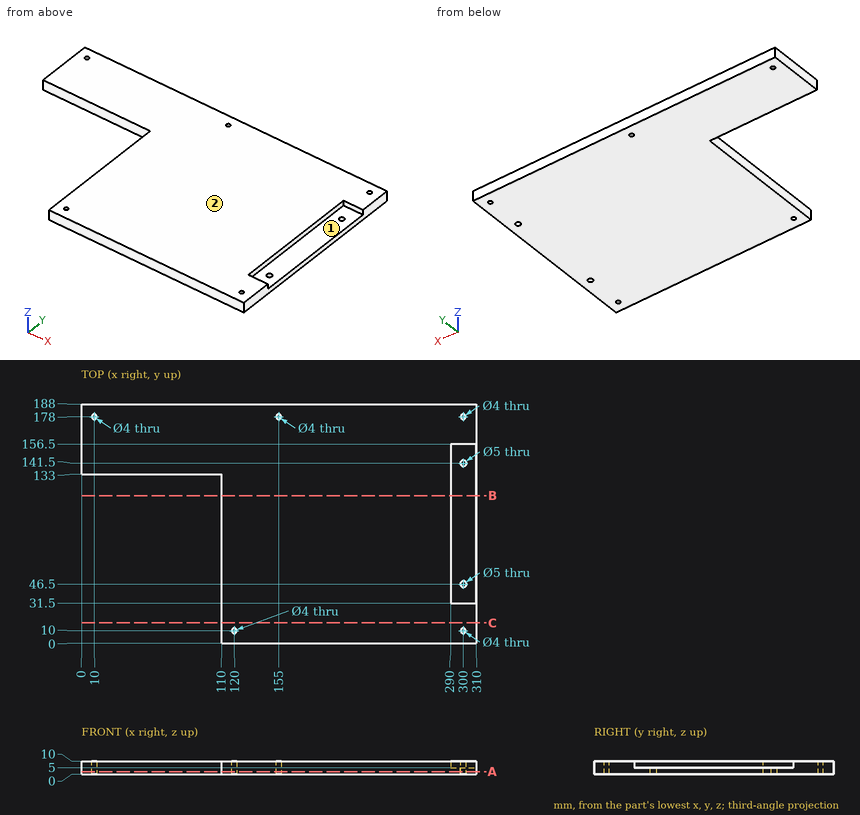
Here's the drawing with two shaded views (mm, measured from the low corner). I have some questions. Give positions to 0.01 mm unless a question says otherwise; leave off trailing zeros. Write each loop counter-clockwise with the first axis right and the second up, starting at its lowest first coordinate (ties: lowest second). Pieces come first, ordered by that corner, then holes. Notation, with made-up numbers: (11.5, 74.5) -> (47.5, 74.5) arc R15 ccw to (47.5, 86.5) -> close; hole circle Ø2 at (10, -15.75). An arc over 180 degrees is marked (long way). Use one line per item in the form item = value. Start each with the question number.
1. Thinking about a two-plate mould opening in Y: for the marked faces 1 and 2, which applies, +Y half, -Y half, draft (parallel to the pull), parting line (faces both ways), or undercut?
2. Imagine slicing it at C-C on y = 16. List the corners of the cut face in (x, z) for me, plus the area to 3 significant figures.
3. If I drill on L1, parallel to Y at x = 300, z = 1.8; L2, parallel to Y at x = 120, z = 3.75; L3, parallel to X at y = 141.5, z = 1.5, over which ranges is the centre line in solid material (lowest first)?
4. Will these pins go through, and if not, where does the flat tip stop? pin 1 Ø3 at (x, y) = (300, 10) entering from +Z; pin 2 Ø2 at (y, z) = (47.5, 2.5) entering from -X; pin 3 Ø10 at (x, y) = (302.5, 73) entering from +Z; pin 4 Ø2.5 at (y, z) = (74, 6.5) entering from +X.
5. Imagine slicing it at A-A on z = 2. List the corners of the cut face in (x, y) for me.
6. Imagine slicing it at B-B on y = 116. List the corners of the cut face in (x, z) for me.
Entries:
q1.face_1 = undercut
q1.face_2 = draft
q2.outline = (110, 0) -> (310, 0) -> (310, 10) -> (110, 10) -> close
q2.area = 2,000 mm²
q3.L1 = 0 to 8, 12 to 44, 49 to 139, 144 to 176, 180 to 188
q3.L2 = 0 to 8, 12 to 188
q3.L3 = 0 to 297.5, 302.5 to 310
q4.pin_1 = through
q4.pin_2 = 110
q4.pin_3 = 5
q4.pin_4 = 290
q5.outline = (0, 133) -> (110, 133) -> (110, 0) -> (310, 0) -> (310, 188) -> (0, 188) -> close; hole circle Ø4 at (10, 178); hole circle Ø4 at (120, 10); hole circle Ø4 at (155, 178); hole circle Ø5 at (300, 46.5); hole circle Ø5 at (300, 141.5); hole circle Ø4 at (300, 10); hole circle Ø4 at (300, 178)
q6.outline = (110, 0) -> (310, 0) -> (310, 5) -> (290, 5) -> (290, 10) -> (110, 10) -> close
